from build123d import *

# Parameters (mm, degrees)
SKETCH1_R           = 35.5
BOSS_EXTRUDE1_DEPTH = 14
CUT_EXTRUDE1_DEPTH  = 24
SKETCH3_W           = 20
SKETCH3_H           = 10
CUT_EXTRUDE2_DEPTH  = 25
SKETCH4_R           = 1.75
CUT_EXTRUDE3_DEPTH  = 58.484780595
CUT_EXTRUDE4_DEPTH  = 3
SKETCH6_R           = 1.75
CUT_EXTRUDE5_DEPTH  = 58.484780595
CUT_EXTRUDE6_DEPTH  = 3
SKETCH8_R           = 7.5
CUT_EXTRUDE7_DEPTH  = 56.646203824


with BuildPart() as part:
    # Sketch1 → Boss-Extrude1 (new, symmetric)
    with BuildSketch(Plane(origin=(0, 0, 0), x_dir=(1, 0, 0), z_dir=(0, 1, 0))):
        with Locations(Location((0, 0, 0), (0, 0, 270))):
            Circle(SKETCH1_R)
    extrude(amount=BOSS_EXTRUDE1_DEPTH, both=True)

    # Sketch2 → Cut-Extrude1 (cut)
    with BuildSketch(Plane(origin=(0, 14, 0), x_dir=(1, 0, 0), z_dir=(0, 1, 0))):
        Polygon((27.2, 27.7), (27.2, 4.7), (22.964840301, -2.635511777), (28.588903685, -5.882566285), (10.388903685, -37.405890983), (-9.529680602, -25.905890983), (-13.764840301, -18.570379206), (-19.388903685, -21.817433715), (-37.588903685, 9.705890983), (-17.670319398, 21.205890983), (-9.2, 21.205890983), (-9.2, 27.7), align=None)
    extrude(amount=-CUT_EXTRUDE1_DEPTH, mode=Mode.SUBTRACT)

    # Sketch3 → Cut-Extrude2 (cut)
    with BuildSketch(Plane(origin=(0, 14, 0), x_dir=(1, 0, 0), z_dir=(0, 1, 0))):
        Polygon((-35.488903685, 6.068584287), (-44.149157723, 1.068584287), (-34.149157723, -16.251923789), (-25.488903685, -11.251923789), align=None)
        with Locations((13, 32.7)):
            Rectangle(SKETCH3_W, SKETCH3_H)
        Polygon((12.488903685, -33.768584287), (21.149157723, -38.768584287), (31.149157723, -21.448076211), (22.488903685, -16.448076211), align=None)
    extrude(amount=-CUT_EXTRUDE2_DEPTH, mode=Mode.SUBTRACT)

    # Sketch4 → Cut-Extrude3 (cut, through all)
    with BuildSketch(Plane(origin=(0, 14, 0), x_dir=(1, 0, 0), z_dir=(0, 1, 0))):
        with Locations(Location((-4.453539231, 31.6885782, 0), (0, 0, 270))):
            Circle(SKETCH4_R)
        with Locations(Location((29.669883346, -11.987410989, 0), (0, 0, 270))):
            Circle(SKETCH4_R)
        with Locations(Location((-25.216344115, -19.70116721, 0), (0, 0, 270))):
            Circle(SKETCH4_R)
    extrude(amount=-CUT_EXTRUDE3_DEPTH, mode=Mode.SUBTRACT)

    # Sketch5 → Cut-Extrude4 (cut)
    with BuildSketch(Plane.XZ.offset(14)):
        Polygon((-26.861792383, 22.55116721), (-28.50724065, 19.70116721), (-26.861792383, 16.85116721), (-23.570895848, 16.85116721), (-21.925447581, 19.70116721), (-23.570895848, 22.55116721), align=None)
        Polygon((32.960779881, 11.987410989), (31.315331613, 14.837410989), (28.024435079, 14.837410989), (26.378986812, 11.987410989), (28.024435079, 9.137410989), (31.315331613, 9.137410989), align=None)
        Polygon((-6.098987498, -34.5385782), (-2.808090964, -34.5385782), (-1.162642696, -31.6885782), (-2.808090964, -28.8385782), (-6.098987498, -28.8385782), (-7.744435765, -31.6885782), align=None)
    extrude(amount=-CUT_EXTRUDE4_DEPTH, mode=Mode.SUBTRACT)

    # Sketch6 → Cut-Extrude5 (cut, through all)
    with BuildSketch(Plane.XZ.offset(14)):
        with Locations(Location((6.619546181, 31.534609691, 0), (0, 0, 270))):
            Circle(SKETCH6_R)
        with Locations(Location((-3.772758664, 25.534609691, 0), (0, 0, 270))):
            Circle(SKETCH6_R)
        with Locations(Location((24, -21.5, 0), (0, 0, 270))):
            Circle(SKETCH6_R)
        with Locations(Location((24, -9.5, 0), (0, 0, 270))):
            Circle(SKETCH6_R)
        with Locations(Location((-30.619546181, -10.034609691, 0), (0, 0, 270))):
            Circle(SKETCH6_R)
        with Locations(Location((-20.227241336, -16.034609691, 0), (0, 0, 270))):
            Circle(SKETCH6_R)
    extrude(amount=-CUT_EXTRUDE5_DEPTH, mode=Mode.SUBTRACT)

    # Sketch7 → Cut-Extrude6 (cut)
    with BuildSketch(Plane.XZ.offset(14)):
        Polygon((9.469546181, 29.889161424), (9.469546181, 33.180057958), (6.619546181, 34.825506225), (3.769546181, 33.180057958), (3.769546181, 29.889161424), (6.619546181, 28.243713156), align=None)
        Polygon((-30.619546181, -6.743713156), (-33.469546181, -8.389161424), (-33.469546181, -11.680057958), (-30.619546181, -13.325506225), (-27.769546181, -11.680057958), (-27.769546181, -8.389161424), align=None)
        Polygon((-23.077241336, -14.389161424), (-23.077241336, -17.680057958), (-20.227241336, -19.325506225), (-17.377241336, -17.680057958), (-17.377241336, -14.389161424), (-20.227241336, -12.743713156), align=None)
        Polygon((-0.922758664, 27.180057958), (-3.772758664, 28.825506225), (-6.622758664, 27.180057958), (-6.622758664, 23.889161424), (-3.772758664, 22.243713156), (-0.922758664, 23.889161424), align=None)
        Polygon((21.15, -23.145448267), (24, -24.790896534), (26.85, -23.145448267), (26.85, -19.854551733), (24, -18.209103466), (21.15, -19.854551733), align=None)
        Polygon((24, -12.790896534), (26.85, -11.145448267), (26.85, -7.854551733), (24, -6.209103466), (21.15, -7.854551733), (21.15, -11.145448267), align=None)
    extrude(amount=-CUT_EXTRUDE6_DEPTH, mode=Mode.SUBTRACT)

    # Sketch8 → Cut-Extrude7 (cut, through all)
    with BuildSketch(Plane(origin=(0, -10, 0), x_dir=(1, 0, 0), z_dir=(0, 1, 0))):
        with Locations(Location((0, 0, 0), (0, 0, 270))):
            Circle(SKETCH8_R)
    extrude(amount=-CUT_EXTRUDE7_DEPTH, mode=Mode.SUBTRACT)


solid = part.part
Read the model definition and answer for the solid it produces. Units are mm, in the model's axes. A direction names the side the tool comes from. Round coordinates to 2 decimals unless told otherwise and drop trailing zeros. Order: outer loops, then holes, each group sorted by start corner. A loop starts at its lowest first (then second) coordinate and runs counter-clockwise, first axis right, second up.
1) Straight lines are drawn through the part: L1, parallel to X at y = 12, z = 19; L2, parallel to Z at x = -3.5, y = -9.75; L3, parallel to Y at x = 22.5, z = 2. For each, find the intervals that lie inside material, in ascending order.
2) The part is cut by section C-C on x = 0. Write down the section's boundary in (y, z), plus the area to 3 significant figures.
3) For faces 4 (the face through (-28.86, 1.68, 13.2)), 5 (the face through (21.15, -13, -9)), 6 (the face through (-3, 2, -27.7)), determine the directions among +Z, -Z, +X, -X, +Y, -Y from which every point of the face is accessible in a straight line to the end or side of a thin tool.
4) The mould has two halves that part along X. Classify faces 1 (the face through (25.11, 2.17, -1.08)), 2 (the face through (-16.538, 2.168, 20.171)), 3 (the face through (-16, 14, 27)): released by +X, released by -X, zero draft, split by the parting line, or undercut.
5) The part is cut by section B-B on z = 0. Write down the section's boundary in (x, y), plus the area to 3 significant figures.
6) The part is cut by section A-A on y = -3. Write down the section's boundary in (x, z), plus the area to 3 significant figures.
7) Flat-ended cylindrical pins translate along their axes: pin 1 (3.5 mm diameter, centred on y = -13, z = -20.5, fed in from +X); pin 2 (3 mm diameter, centred on x = 26, z = 24, fed in from +Y); pin 3 (1 mm diameter, centred on x = -7.5, y = 1, fed in from -Z); pin 4 (4.5 mm diameter, centred on x = -5.5, z = -30.5, fed in from -Y). Find the tip coordinate at first contact, or state that the pin passes through.
8) The part is cut by section D-D on x = 17. Write down the section's boundary in (y, z), plus the area to 3 significant figures.
Resolved:
1. L1: x = -29.99 to -26.82, -23.61 to -21.02, -14.51 to -13.52, 26.91 to 29.99
1. L2: z = -35.33 to -33.16, -30.22 to -27.7, 29.39 to 35.33
1. L3: y = -14 to -10
2. outline: (-14, -35.5) - (14, -35.5) - (14, -27.7) - (-10, -27.7) - (-10, -7.5) - (-14, -7.5) - close; (-14, 7.5) - (-10, 7.5) - (-10, 31.41) - (14, 31.41) - (14, 35.5) - (-14, 35.5) - close
2. area: 509 mm2
3. face 4: -X, +Y
3. face 5: -Y
3. face 6: +X, +Y
4. face 1: released by -X
4. face 2: undercut
4. face 3: zero draft
5. outline: (-35.5, -14) - (-7.5, -14) - (-7.5, -10) - (-31.99, -10) - (-31.99, -11) - (-35.5, -11) - close; (7.5, -14) - (35.5, -14) - (35.5, 14) - (24.49, 14) - (24.49, -10) - (7.5, -10) - close
5. area: 485 mm2
6. outline: (-33.36, -12.15) arc R35.5 ccw to (3, -35.37) - (3, -27.7) - (-9.2, -27.7) - (-9.2, -21.21) - (-17.67, -21.21) - close; (-32.13, 15.09) - (-25.49, 11.25) - (-19.39, 21.82) - (-13.76, 18.57) - (-9.53, 25.91) - (6.16, 34.96) arc R35.5 ccw to start; (22.49, 16.45) - (28.59, 5.88) - (22.96, 2.64) - (27.2, -4.7) - (27.2, -22.81) arc R35.5 ccw to (29.13, 20.28) - close; hole circle Ø3.5 at (-25.22, 19.7); hole circle Ø3.5 at (-4.45, -31.69); hole circle Ø3.5 at (29.67, 11.99)
6. area: 870 mm2
7. pin 1: stops at x = 30.14
7. pin 2: stops at y = -11
7. pin 3: stops at z = -34.8
7. pin 4: stops at y = -14
8. outline: (-14, -31.16) - (-11, -31.16) - (-11, -27.7) - (-10, -27.7) - (-10, 25.96) - (-11, 25.96) - (-11, 31.16) - (-14, 31.16) - close
8. area: 241 mm2
